Build history of the part. All positions in model axes, mm. A direction names the side the tool comes from. Give positions to 0.01 mm unless a question says otherwise; leave off trailing zeros. Loops run counter-clockwise (first coordinate to the right, second up) from the corner with the lowest first, then second, coordinate; pieces in that order, holes last.
1) Band-saw the part on A-A on z = 0. List the corners of the cut face in (x, y), then the cut area to 4 significant figures.
2) Two-plate mould, pull along X, no slides. Class faces 4 (the cylindrical face through (23.594, -0.74, -0.889)), 5 (the flat face through (20, 0, 3)), 6 (the cylindrical face through (0.57, -0.74, 11.9)): +X half, -X half, draft (parallel to the pull), parting line (faces both ways), or undercut.
3) Wall check: line 1 (X direction, y = -0.85, z = -8.5); line 2 (Y direction, x = 30.5, z = 5); line 3 (Z direction, x = 28, y = -33). Give the ranges that are in metal, low to high.
4) Band-saw the part on D-D on z = -8.5. List the corners of the cut face in (x, y).
5) 3-axis set-ups, long thin cutter, end or side, ignore diameter. For faces 1 (the flat face through (7, -1, 12.5)), 2 (the flat face through (20, -1.5, 3)), 3 (the cylindrical face through (38.25, -43.03, 20.74)): which of +Z, -Z, +X, -X, +Y, -Y reach the whole face in a straight line?
6) Band-saw the part on B-B on x = 18.3. List the corners of the cut face in (y, z), then the cut area to 3 significant figures.
7) Band-saw the part on C-C on y = -42. List the corners of the cut face in (x, z), then the cut area to 3 significant figures.
8) Flat gauge pins, fed straight in: P1, Ø5.5, axis at y = -18.5, z = 17.5, coming from the -X side; P2, Ø6, axis at x = 12.5, y = -28, coming from the -Z side; P3, Ø3, axis at x = 8, z = 8.5, coming from the -Y side; P4, Ø8, axis at x = 30.5, z = -7.5, coming from the -Y side. Where does each tip first touch, or does it go through?
```python
from build123d import *

# Parameters (mm, degrees)
SKETCH1_W            = 41.6
SKETCH1_H            = 1.5
BASE_FLANGE1_DEPTH   = 12.5
M3_CLEARANCE_HOLE2_D = 3.4
M3_CLEARANCE_HOLE3_D = 3.4
SKETCH12_R           = 5.1
SKETCH12_R_2         = 4.1
CUT_EXTRUDE1_DEPTH   = 1.5
EDGE_FLANGE1_DEPTH   = 25
SKETCH22_W           = 1.5
SKETCH22_H           = 25
CUT_EXTRUDE2_DEPTH   = 1.5
FILLET1_R            = 2
M3_CLEARANCE_HOLE4_D = 3.4


# Sheet-metal steps are written as plain solids
with BuildPart() as part:
    # Sketch1 → Base-Flange1 (new, symmetric)
    with BuildSketch(Plane.XY):
        with Locations((20.8, -0.75)):
            Rectangle(SKETCH1_W, SKETCH1_H)
    extrude(amount=BASE_FLANGE1_DEPTH, both=True)

    # M3 Clearance Hole2 (through all)
    with Locations(Plane(origin=(0, -1.5, 0), x_dir=(-1, 0, 0), z_dir=(0, -1, 0))):
        with Locations((-8, -8.5), (-8, 8.5)):
            Hole(M3_CLEARANCE_HOLE2_D / 2)

    # M3 Clearance Hole3 (through all)
    with Locations(Plane(origin=(0, -1.5, 0), x_dir=(-1, 0, 0), z_dir=(0, -1, 0))):
        with Locations((-24.422, -5.499261314), (-33.947, 0), (-24.422, 5.499261314)):
            Hole(M3_CLEARANCE_HOLE3_D / 2)

    # Sketch12 → Cut-Extrude1 (cut)
    with BuildSketch(Plane(origin=(0, 0, 0), x_dir=(1, 0, 0), z_dir=(0, 1, 0))):
        with Locations(Location((8, 0, 0), (0, 0, 270))):
            Circle(SKETCH12_R)
        with Locations(Location((27.597, 0, 0), (0, 0, 270))):
            Circle(SKETCH12_R_2)
    extrude(amount=-CUT_EXTRUDE1_DEPTH, mode=Mode.SUBTRACT)

    # Edge-Flange1 section (across the edge) → Edge-Flange1 (add)
    with BuildSketch(Plane(origin=(40.1, -1.5, 20), x_dir=(0, 0, -1), z_dir=(-1, 0, 0))):
        with BuildLine():
            Line((-1.5, 1.5), (-1.5, 45.5))
            Line((-1.5, 45.5), (0, 45.5))
            Line((0, 45.5), (0, 1.5))
            ThreePointArc((0, 1.5), (0.439339828, 0.439339828), (1.5, 0))
            Line((1.5, 0), (7.5, 0))
            Line((7.5, 0), (7.5, -1.5))
            Line((7.5, -1.5), (1.5, -1.5))
            ThreePointArc((1.5, -1.5), (-0.621320344, -0.621320344), (-1.5, 1.5))
        make_face()
    extrude(amount=EDGE_FLANGE1_DEPTH)

    # Sketch22 → Cut-Extrude2 (cut)
    with BuildSketch(Plane(origin=(0, 0, 0), x_dir=(1, 0, 0), z_dir=(0, 1, 0))):
        with Locations((40.85, 0)):
            Rectangle(SKETCH22_W, SKETCH22_H)
    extrude(amount=-CUT_EXTRUDE2_DEPTH, mode=Mode.SUBTRACT)

    # Fillet1
    fillet1_edges = [part.edges().sort_by_distance(p)[0] for p in [
        (0, -0.75, 12.5),
        (0, -0.75, -12.5),
        (15.1, -0.75, 12.5),
        (40.1, -47, 20.75),
        (15.1, -47, 20.75),
        (40.1, -0.75, -12.5),
    ]]
    fillet(fillet1_edges, radius=FILLET1_R)

    # M3 Clearance Hole4 (through all)
    with Locations(Plane.XY.offset(21.5)):
        with Locations((36.9, -42), (18.3, -42)):
            Hole(M3_CLEARANCE_HOLE4_D / 2)


solid = part.part
```
Findings below:
1. outline: (0, -1.5) - (2.9, -1.5) - (2.9, 0) - (0, 0) - close; (13.1, -1.5) - (23.5, -1.5) - (23.5, 0) - (13.1, 0) - close; (31.7, -1.5) - (32.25, -1.5) - (32.25, 0) - (31.7, 0) - close; (35.65, -1.5) - (40.1, -1.5) - (40.1, 0) - (35.65, 0) - close
1. area: 27.45 mm2
2. face 4: undercut
2. face 5: draft
2. face 6: -X half
3. line 1: x = 0 to 6.3, 9.7 to 40.1
3. line 2: y = -1.5 to 0
3. line 3: z = 20 to 21.5
4. outline: (0, -1.5) - (6.3, -1.5) - (6.3, 0) - (0, 0) - close; (9.7, -1.5) - (40.1, -1.5) - (40.1, 0) - (9.7, 0) - close
5. face 1: +Z, -X, +Y, -Y
5. face 2: -Z, +X, -X, -Y
5. face 3: +Z, -Z
6. outline: (-47, 20) - (-43.7, 20) - (-43.7, 21.5) - (-47, 21.5) - close; (-40.3, 20) - (-3, 20) arc R1.5 cw to (-1.5, 18.5) - (-1.5, -12.5) - (0, -12.5) - (0, 18.5) arc R3 ccw to (-3, 21.5) - (-40.3, 21.5) - close
6. area: 113 mm2
7. outline: (15.1, 20) - (16.6, 20) - (16.6, 21.5) - (15.1, 21.5) - close; (20, 20) - (35.2, 20) - (35.2, 21.5) - (20, 21.5) - close; (38.6, 20) - (40.1, 20) - (40.1, 21.5) - (38.6, 21.5) - close
7. area: 27.3 mm2
8. P1: stops at x = 15.1
8. P2: stops at z = 20
8. P3: passes through
8. P4: stops at y = -1.5
